Source: CAD feature listing. Evaluate the final solid. Frame: model axes, mm. Coordinates: 2 decimals unless noted, no trailing zeros. Write each loop counter-clockwise with the first axis right and the second up, starting at its lowest first coordinate (ties: lowest second). Pieces come first, ordered by that corner, then holes. Notation, with made-up numbers: (-33.5, -8.75) - (24.5, -8.75) arc R18 ccw to (24.5, 15.25) - close; hole circle Ø2 at (-16.75, 14). An arc over 180 degrees is marked (long way). One line per item, written item: value.
from build123d import *

# Parameters (mm, degrees)
F0_R     = 2
F1_DEPTH = 4
F2_R     = 0.5
F3_SIZE  = 2


with BuildPart() as f1:
    # F0 (on Top) → F1 (new body)
    with BuildSketch(Plane.XY):
        Polygon((0, -5), (10, -5), (10, 5), (0, 5), (-10, 5), (-10, -5), align=None)
        with Locations((-5, 0)):
            Circle(F0_R, mode=Mode.SUBTRACT)
        with Locations((5, 0)):
            Circle(F0_R, mode=Mode.SUBTRACT)
    extrude(amount=F1_DEPTH)

    # F2
    f2_edges = [f1.edges().sort_by_distance(p)[0] for p in [
        (0, -5, 4),
        (-10, 0, 4),
        (0, 5, 4),
        (10, 0, 4),
        (-10, 0, 0),
        (0, -5, 0),
        (10, 0, 0),
        (0, 5, 0),
    ]]
    fillet(f2_edges, radius=F2_R)

    # F3
    f3_edges = [f1.edges().sort_by_distance(p)[0] for p in [
        (3, 0, 4),
        (-7, 0, 4),
    ]]
    chamfer(f3_edges, length=F3_SIZE)


solid = f1.part
1) Material intervals for line 1 (Y direction, x = 5, z = 0.65); line 2 (X direction, y = -1.5, z = 1); line 3 (X direction, y = -0.5, z = 0.55), sorted ascending.
Values found:
line 1: -5 to -2, 2 to 5
line 2: -10 to -6.32, -3.68 to 3.68, 6.32 to 10
line 3: -10 to -6.94, -3.06 to 3.06, 6.94 to 10
2) Section query B-B on x = -5. Output: boundary loops of the cut face in (y, z), then the cut area to 3 significant figures.
Values found:
outline: (-5, 0.5) arc R0.5 ccw to (-4.5, 0) - (-2, 0) - (-2, 2) - (-4, 4) - (-4.5, 4) arc R0.5 ccw to (-5, 3.5) - close; (2, 0) - (4.5, 0) arc R0.5 ccw to (5, 0.5) - (5, 3.5) arc R0.5 ccw to (4.5, 4) - (4, 4) - (2, 2) - close
area: 19.8 mm2
3) Draft query along Y for faces 1 (the flat face through (0, 5, 2)), 2 (the cylindrical face through (-6.6, -1.2, 1)), 3 (the flat face through (0, 0, 4)). Return one class per face: released by +Y, released by -Y, zero draft, split by the parting line, or undercut.
Values found:
face 1: released by +Y
face 2: undercut
face 3: zero draft
4) Section query D-D on z = 2.85. Output: boundary loops of the cut face in (x, y).
Values found:
outline: (-10, -5) - (10, -5) - (10, 5) - (-10, 5) - close; hole circle Ø5.7 at (-5, 0); hole circle Ø5.7 at (5, 0)
5) Section query A-A on y = 0. Output: boundary loops of the cut face in (x, z).
Values found:
outline: (-10, 0.5) arc R0.5 ccw to (-9.5, 0) - (-7, 0) - (-7, 2) - (-9, 4) - (-9.5, 4) arc R0.5 ccw to (-10, 3.5) - close; (-3, 0) - (3, 0) - (3, 2) - (1, 4) - (-1, 4) - (-3, 2) - close; (7, 0) - (9.5, 0) arc R0.5 ccw to (10, 0.5) - (10, 3.5) arc R0.5 ccw to (9.5, 4) - (9, 4) - (7, 2) - close
6) Section query C-C on z = 1.05. Output: boundary loops of the cut face in (x, y), then the cut area to 3 significant figures.
Values found:
outline: (-10, -5) - (10, -5) - (10, 5) - (-10, 5) - close; hole circle Ø4 at (-5, 0); hole circle Ø4 at (5, 0)
area: 175 mm2
